Here's how the part is built. I have some questions about the finished solid (model axes, mm). A direction names the side the tool comes from. Coordinates: 2 decimals unless noted, no trailing zeros. Write each loop counter-clockwise with the first axis right and the second up, starting at its lowest first coordinate (ties: lowest second). Pieces come first, ordered by that corner, then holes.
Item 1: For faces 1 (the face through (9.25, 30, 1)), 2 (the face through (40, 60, 1)), 3 (the face through (-28, 71, 1)), which set-ups out of +Z, -Z, +X, -X, +Y, -Y let a thin tool reach every point of the face, with its end or its side?
Item 2: If I drill on line 1 (Y direction, x = 40, z = 2.1); line 2 (X direction, y = 49, z = 1.25); line 3 (X direction, y = 28.5, z = 2.15), over which ranges is the centre line in solid material (lowest first)?
Item 3: If we section it at C-C (y = 28): Please give me the cut outline in (x, z).
Item 4: If we section it at A-A (x = -40): Please give me the cut outline in (y, z).
Item 5: If we section it at D-D (z = 1.6): Count the separate pieces of the cut face and the enclosed holes in it, then the cut area to 3 significant figures.
Item 6: I'm going to push flat-ended pins straight in: pin 1 Ø1 at (x, z) = (-37, 0.5) entering from +Y; pin 2 Ø1.5 at (y, z) = (71, 1.5) entering from -X; pin 3 Ø0.9 at (y, z) = (72.5, 2) entering from +X. Where does each tip first touch, or does it pass through?
Item 7: We'd pull the mould along X, two halves only. Please class faces 4 (the face through (50, 30, 1)), 5 (the face through (-39, 60, 1)), 6 (the face through (-8.48, 19.43, 1.52)): +X half, -X half, draft (parallel to the pull), parting line (faces both ways), or undercut.
Item 8: If we section it at B-B (y = 15): Please give me the cut outline in (x, z), then the cut area to 3 significant figures.
from build123d import *

# Parameters (mm, degrees)
EXTRUDE_1_DEPTH     = 3
SKETCH_2_R          = 1.55
CUT_EXTRUDE_1_DEPTH = 95.387499172
FILLET_1_R          = 1
SKETCH_3_R          = 2.55
CUT_EXTRUDE_2_DEPTH = 95.387499172
SKETCH_4_R          = 1.55
CUT_EXTRUDE_3_DEPTH = 95.387499172


with BuildPart() as part:
    # ｽｹｯﾁ1 → ﾎﾞｽ - 押し出し1 (new body)
    with BuildSketch(Plane.XY):
        Polygon((-28, 80), (-28, 60), (-50, 60), (-50, 0), (50, 0), (50, 60), (28, 60), (28, 80), align=None)
        with BuildLine():
            Line((-9.25, 34.415880433), (-9.25, 25.584119567))
            ThreePointArc((-9.25, 25.584119567), (0, 19.75), (9.25, 25.584119567))
            Line((9.25, 25.584119567), (9.25, 34.415880433))
            ThreePointArc((9.25, 34.415880433), (0, 40.25), (-9.25, 34.415880433))
        make_face(mode=Mode.SUBTRACT)
    extrude(amount=EXTRUDE_1_DEPTH)

    # ｽｹｯﾁ2 → ｶｯﾄ - 押し出し1 (cut, through all)
    with BuildSketch(Plane.XY.offset(3)):
        with Locations((-9.192388155, 39.192388155)):
            Circle(SKETCH_2_R)
        with Locations((9.192388155, 39.192388155)):
            Circle(SKETCH_2_R)
        with Locations((9.192388155, 20.807611845)):
            Circle(SKETCH_2_R)
        with Locations((-9.192388155, 20.807611845)):
            Circle(SKETCH_2_R)
    extrude(amount=-CUT_EXTRUDE_1_DEPTH, mode=Mode.SUBTRACT)

    # ﾌｨﾚｯﾄ1
    fillet_1_edges = [part.edges().sort_by_distance(p)[0] for p in [
        (28, 60, 1.5),
        (-28, 60, 1.5),
    ]]
    fillet(fillet_1_edges, radius=FILLET_1_R)

    # ｽｹｯﾁ3 → ｶｯﾄ - 押し出し2 (cut, through all)
    with BuildSketch(Plane.XY.offset(3)):
        with Locations((-40, 50)):
            Circle(SKETCH_3_R)
        with Locations(Location((-40, 10, 0), (0, 0, 180))):
            Circle(SKETCH_3_R)
        with Locations((40, 10)):
            Circle(SKETCH_3_R)
        with Locations(Location((40, 50, 0), (0, 0, 180))):
            Circle(SKETCH_3_R)
    extrude(amount=-CUT_EXTRUDE_2_DEPTH, mode=Mode.SUBTRACT)

    # ｽｹｯﾁ4 → ｶｯﾄ - 押し出し3 (cut, through all)
    with BuildSketch(Plane.XY.offset(3)):
        with Locations((25, 45)):
            Circle(SKETCH_4_R)
        with Locations((25, 15)):
            Circle(SKETCH_4_R)
        with Locations((-25, 15)):
            Circle(SKETCH_4_R)
        with Locations((-25, 45)):
            Circle(SKETCH_4_R)
    extrude(amount=-CUT_EXTRUDE_3_DEPTH, mode=Mode.SUBTRACT)


solid = part.part
Answer list:
1. face 1: +Z, -Z
1. face 2: +Z, -Z, +X, +Y
1. face 3: +Z, -Z, -X, +Y
2. line 1: y = 0 to 7.45, 12.55 to 47.45, 52.55 to 60
2. line 2: x = -50 to -42.35, -37.65 to 37.65, 42.35 to 50
2. line 3: x = -50 to -9.25, 9.25 to 50
3. outline: (-50, 0) - (-9.25, 0) - (-9.25, 3) - (-50, 3) - close; (9.25, 0) - (50, 0) - (50, 3) - (9.25, 3) - close
4. outline: (0, 0) - (7.45, 0) - (7.45, 3) - (0, 3) - close; (12.55, 0) - (47.45, 0) - (47.45, 3) - (12.55, 3) - close; (52.55, 0) - (60, 0) - (60, 3) - (52.55, 3) - close
5. separate pieces: 1
5. enclosed holes: 13
5. area: 6,660 mm2
6. pin 1: stops at y = 60
6. pin 2: stops at x = -28
6. pin 3: stops at x = 28
7. face 4: +X half
7. face 5: draft
7. face 6: undercut
8. outline: (-50, 0) - (-26.55, 0) - (-26.55, 3) - (-50, 3) - close; (-23.45, 0) - (23.45, 0) - (23.45, 3) - (-23.45, 3) - close; (26.55, 0) - (50, 0) - (50, 3) - (26.55, 3) - close
8. area: 281 mm2
